Verification items for this drawing (mm, ordinates from the low corner). A direction names the side the tool comes from. Give positions to 0.01 mm unless a question says otherwise; leave off trailing zeros. Loops run counter-clockwise (first coordinate to the right, second up) from the corner with the lowest first, then second, coordinate; pieces in that order, holes last. Notation, with made-up numbers: (60, 8.25) -> (87, 8.25) arc R11 cw to (87, 26.25) -> close; hole circle Ø9 at (-3.5, 18.25). An arc over 180 degrees is marked (long way). Answer in a Markdown table with one row per item. Add a question column.
Q1. Gauge pin test, flat ends, axial feed: P1, Ø1.5, axis at x = 1, y = 4.5, coming from the -Z side; P2, Ø1.6, axis at x = 2, z = 0.5, coming from the -Y side. Record the tip position at first contact, or that the pin passes through.
Q2. Section check A-A on z = 1.4. Enter the section's corners in (x, y).
Q3. Section check C-C on y = 5.5. Enter the section's corners in (x, z), and give its area (3 significant figures).
Q4. Section check B-B on x = 1.4. Enter the section's corners in (y, z).
Q5. Set-up check for the marked faces 1 and 2: record each of +Z, -Z, +X, -X, +Y, -Y from which the full face is reachable in a straight line by a thin tool's end or side.
Q6. Material ranges on probe 1 along Y at (x, z) = (2.05, 0.45); probe 2 along Z at (x, y) = (1.25, 4.5), recorded low to high.
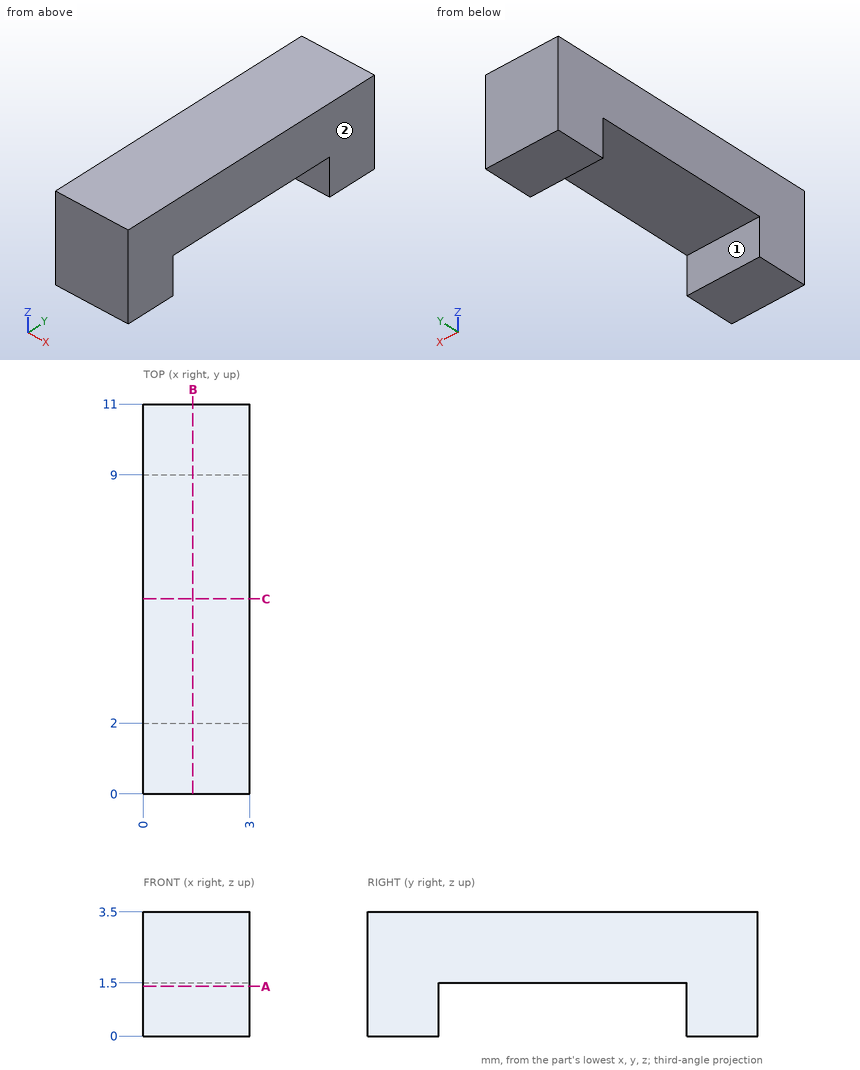
Taken from the geometry:
| question | item | result |
|---|---|---|
| 1 | P1 | stops at z = 1.5 |
| 1 | P2 | stops at y = 0 |
| 2 | outline | (0, 0) -> (3, 0) -> (3, 2) -> (0, 2) -> close; (0, 9) -> (3, 9) -> (3, 11) -> (0, 11) -> close |
| 3 | outline | (0, 1.5) -> (3, 1.5) -> (3, 3.5) -> (0, 3.5) -> close |
| 3 | area | 6.00 mm² |
| 4 | outline | (0, 0) -> (2, 0) -> (2, 1.5) -> (9, 1.5) -> (9, 0) -> (11, 0) -> (11, 3.5) -> (0, 3.5) -> close |
| 5 | face 1 | -Z, +X, -X |
| 5 | face 2 | +Z, -Z, +X, +Y, -Y |
| 6 | probe 1 | y = 0 to 2, 9 to 11 |
| 6 | probe 2 | z = 1.5 to 3.5 |
